Verification items for the finished model (mm, model axes). A direction names the side the tool comes from. Round coordinates to 2 decimals unless told otherwise and drop trailing zeros. Order: outer loops, then holes, each group sorted by start corner. A loop starts at its lowest first (then second) coordinate and runs counter-clockwise, first axis right, second up. Notation, with made-up numbers: (34.5, -19.5) -> (90.5, -19.5) arc R16 cw to (90.5, -14.5) -> close; hole circle Ø6 at (50, -9.5). An arc over 180 degrees is marked (long way). Put each result on its own line as item: value.
```python
from build123d import *

# Parameters (mm, degrees)
F1_DEPTH = 101.6


with BuildPart() as f1:
    # F0 (on Right) → F1 (new body)
    with BuildSketch(Plane.YZ):
        Polygon((-609.6, 128.40195), (-537.757951, 56.559901), (-394.073853, 56.559901), (-609.6, 272.086048), align=None)
        Polygon((-537.757951, 56.559901), (-609.6, 56.559901), (-609.6, -45.040099), (0, -45.040099), (0, 56.559901), (-394.073853, 56.559901), align=None)
        Polygon((609.6, 272.086048), (394.073853, 56.559901), (537.757951, 56.559901), (609.6, 128.40195), align=None)
        Polygon((0, 56.559901), (0, -45.040099), (609.6, -45.040099), (609.6, 56.559901), (537.757951, 56.559901), (394.073853, 56.559901), align=None)
    extrude(amount=F1_DEPTH)


solid = f1.part
```
Item 1: Sectioned sample at C-C, the plane y = 341.5. Record the boundary of the cut face in (x, z), then the cut area to 3 significant figures.
Geometry check:
outline: (0, -45.04) -> (101.6, -45.04) -> (101.6, 56.56) -> (0, 56.56) -> close
area: 10,300 mm2
Item 2: Tool access check on faces 1 (the face through (50.1, 573.2, 92)), 2 (the face through (50.089, 503.346, 165.832)), 3 (the face through (50, -609.6, 201)). Record the directions out of +Z, -Z, +X, -X, +Y, -Y that give a thin tool (end or side, any length) a straight path to the whole face; none if there is none.
Geometry check:
face 1: +X, -X, +Y
face 2: +Z, +X, -X
face 3: +Z, -Z, +X, -X, -Y
Item 3: Sectioned sample at B-B, the plane x = 66.5. Record the boundary of the cut face in (y, z).
Geometry check:
outline: (-609.6, -45.04) -> (609.6, -45.04) -> (609.6, 56.56) -> (537.76, 56.56) -> (609.6, 128.4) -> (609.6, 272.09) -> (394.07, 56.56) -> (-394.07, 56.56) -> (-609.6, 272.09) -> (-609.6, 128.4) -> (-537.76, 56.56) -> (-609.6, 56.56) -> close
Item 4: Sectioned sample at A-A, the plane z = 235.5. Record the boundary of the cut face in (x, y), then the cut area to 3 significant figures.
Geometry check:
outline: (0, -609.6) -> (101.6, -609.6) -> (101.6, -573.01) -> (0, -573.01) -> close; (0, 573.01) -> (101.6, 573.01) -> (101.6, 609.6) -> (0, 609.6) -> close
area: 7,430 mm2
Item 5: Material ranges on line 1 along Z through (x, y) = (84.5, 376); line 2 along Y through (x, z) = (72.5, 77); line 3 along Y through (x, z) = (27, 139), recorded low to high.
Geometry check:
line 1: -45.04 to 56.56
line 2: -558.2 to -414.51, 414.51 to 558.2
line 3: -609.6 to -476.51, 476.51 to 609.6
Item 6: Release check for a two-part mould opening along Y. For faces 4 (the face through (50.1, -574.2, 93)), 5 (the face through (101.6, -9, 45)), 6 (the face through (50.089, -500.328, 162.814)), 7 (the face through (50, 6, 56.56)) record: pulls with the +Y half, pulls with the -Y half, needs draft (parallel to the pull), parting line crosses it, or undercut.
Geometry check:
face 4: pulls with the -Y half
face 5: needs draft
face 6: undercut
face 7: undercut
Item 7: Sectioned sample at D-D, the plane z = 106.5. Record the boundary of the cut face in (x, y), then the cut area to 3 significant figures.
Geometry check:
outline: (0, -587.7) -> (101.6, -587.7) -> (101.6, -444.01) -> (0, -444.01) -> close; (0, 444.01) -> (101.6, 444.01) -> (101.6, 587.7) -> (0, 587.7) -> close
area: 29,200 mm2
